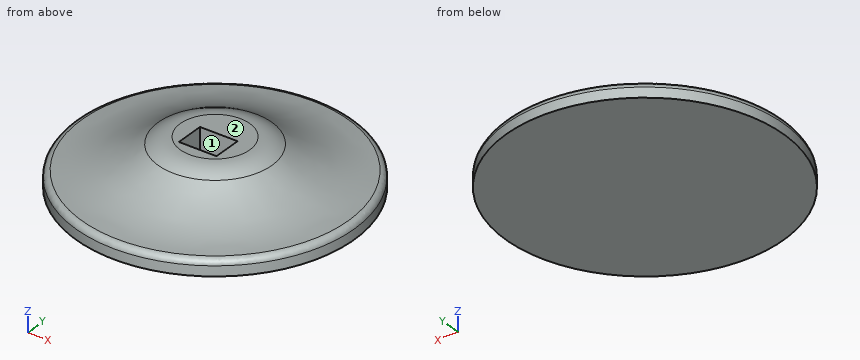
```python
from build123d import *

# Parameters (mm, degrees)
F0_W     = 17.5
F0_H     = 2
F2_W     = 4
F2_H     = 4
F3_DEPTH = 4
F4_R     = 0.75
F5_SCALE = 0.9
F6_DEPTH = 0.33
F7_DEPTH = 0.33
F8_DEPTH = 0.33


with BuildPart() as f1:
    # F0 (on Right) → F1 (revolve)
    with BuildSketch(Plane.YZ):
        with BuildLine():
            Line((0, 1), (17.5, 1))
            ThreePointArc((17.5, 1), (12.0974696672, 1.8050013115), (7.164313392, 4.1500664011))
            ThreePointArc((7.164313392, 4.1500664011), (5.8332762858, 4.7827989716), (4.3755952516, 5))
            Line((4.3755952516, 5), (0, 5))
            Line((0, 5), (0, 1))
        make_face()
        with Locations((8.75, 0)):
            Rectangle(F0_W, F0_H)
    revolve(axis=Axis((0, 0, 2), (0, 0, 1)))

    # F2 (on face) → F3 (cut)
    with BuildSketch(Plane.XY.offset(5)):
        with Locations((0, -1)):
            Rectangle(F2_W, F2_H)
    extrude(amount=-F3_DEPTH, mode=Mode.SUBTRACT)

    # F4
    f4_edges = [f1.edges().sort_by_distance(p)[0] for p in [
        (0, -17.5, 1),
    ]]
    fillet(f4_edges, radius=F4_R)


with BuildPart() as f1_1:
    # F5: moved
    add(f1.part.scale(F5_SCALE))

    # F6 (cut): a face of the model
    f6_faces = [f1_1.faces().sort_by_distance(p)[0] for p in [
        (-1.8, -0.9, 2.7),
    ]]
    extrude(f6_faces, amount=-F6_DEPTH, mode=Mode.SUBTRACT)

    # F7 (cut): a face of the model
    f7_faces = [f1_1.faces().sort_by_distance(p)[0] for p in [
        (1.8, -0.9, 2.7),
    ]]
    extrude(f7_faces, amount=-F7_DEPTH, mode=Mode.SUBTRACT)

    # F8 (add): a face of the model
    f8_faces = [f1_1.faces().sort_by_distance(p)[0] for p in [
        (0, 0.9, 2.7),
    ]]
    extrude(f8_faces, amount=F8_DEPTH)


solid = f1_1.part
```
Here's how the part is built. I have some questions about the finished solid (model axes, mm). Face numbers are marked on the shaded views. Coordinates: 2 decimals unless noted, no trailing zeros. Use a Markdown table: item, result. Add a question column.
(1) We'd pull the mould along Y, two halves only. Please class the marked faces 1 and 2: +Y half, -Y half, draft (parallel to the pull), parting line (faces both ways), or undercut.
(2) I'm going to push flat-ended pins straight in: P1, Ø4, axis at x = 7.5, y = -2.5, coming from the +Z side; P2, Ø1, axis at y = -4, z = 0, coming from the -X side; P3, Ø1, axis at y = 0, z = 3, coming from the -X side. Where does each tip first touch, or does it pass through?
(3) Please list where these lines run through material, in increasing order: line 1 (Z direction, x = -3, y = -9); line 2 (Y direction, x = -0.5, z = -0.15); line 3 (Y direction, x = -5.5, z = -0.05).
Outcome:
| question | item | result |
|---|---|---|
| 1 | face 1 | undercut |
| 1 | face 2 | draft |
| 2 | P1 | stops at z = 4.05 |
| 2 | P2 | stops at x = -15.36 |
| 2 | P3 | stops at x = -8.62 |
| 3 | line 1 | z = -0.9 to 2.12 |
| 3 | line 2 | y = -15.74 to 15.74 |
| 3 | line 3 | y = -14.76 to 14.76 |
